from build123d import *

# Parameters (mm, degrees)
SKETCH1_R                = 2.5
BASE_EXTRUDE_DEPTH       = 1
PROCESS_BENDS1_START     = 0.384624116
PROCESS_BENDS1_OUTLINE_W = 60
PROCESS_BENDS1_OUTLINE_H = 1
PROCESS_BENDS1_DEPTH     = 29.615375884
PROCESS_BENDS1_START_2   = -1.84192973
PROCESS_BENDS1_2_DEPTH   = 3.226553846
PROCESS_BENDS1_START_3   = -30
PROCESS_BENDS1_3_DEPTH   = 61
PROCESS_BENDS1_4_DEPTH   = 60


with BuildPart() as part:
    # Sketch1 → Base-Extrude (new body)
    with BuildSketch(Plane.XY):
        with BuildLine():
            Line((14, 18.25), (28, 18.25))
            ThreePointArc((28, 18.25), (29.414213562, 18.835786438), (30, 20.25))
            Line((30, 20.25), (30, 20.725859478))
            ThreePointArc((30, 20.725859478), (29.686782892, 21.800458695), (28.845236523, 22.538475052))
            Line((28.845236523, 22.538475052), (13.245791834, 29.812615574))
            ThreePointArc((13.245791834, 29.812615574), (12.833434539, 29.952592014), (12.400555311, 30))
            Line((12.400555311, 30), (-286, 30))
            ThreePointArc((-286, 30), (-288.828427125, 28.828427125), (-290, 26))
            Line((-290, 26), (-290, -26))
            ThreePointArc((-290, -26), (-288.828427125, -28.828427125), (-286, -30))
            Line((-286, -30), (12.400555311, -30))
            ThreePointArc((12.400555311, -30), (12.833434539, -29.952592014), (13.245791834, -29.812615574))
            Line((13.245791834, -29.812615574), (28.845236523, -22.538475052))
            ThreePointArc((28.845236523, -22.538475052), (29.686782892, -21.800458695), (30, -20.725859478))
            Line((30, -20.725859478), (30, -20.25))
            ThreePointArc((30, -20.25), (29.414213562, -18.835786438), (28, -18.25))
            Line((28, -18.25), (14, -18.25))
            ThreePointArc((14, -18.25), (8.75, -13), (14, -7.75))
            Line((14, -7.75), (28, -7.75))
            ThreePointArc((28, -7.75), (29.414213562, -7.164213562), (30, -5.75))
            Line((30, -5.75), (30, 5.75))
            ThreePointArc((30, 5.75), (29.414213562, 7.164213562), (28, 7.75))
            Line((28, 7.75), (14, 7.75))
            ThreePointArc((14, 7.75), (8.75, 13), (14, 18.25))
        make_face()
        with Locations((-283, 0)):
            Circle(SKETCH1_R, mode=Mode.SUBTRACT)
    extrude(amount=BASE_EXTRUDE_DEPTH)

    # Process-Bends1: read off the stored shape, not the designer's step
    # Process-Bends1 outline → Process-Bends1 (cut)
    with BuildSketch(Plane.YZ.offset(PROCESS_BENDS1_START)):
        with Locations((0, 0.5)):
            Rectangle(PROCESS_BENDS1_OUTLINE_W, PROCESS_BENDS1_OUTLINE_H)
    extrude(amount=PROCESS_BENDS1_DEPTH, mode=Mode.SUBTRACT)

    # Process-Bends1 2 outline → Process-Bends1 2 (add)
    with BuildSketch(Plane.YZ.offset(PROCESS_BENDS1_START_2)):
        with BuildLine():
            ThreePointArc((18.25, 15.384624116), (13, 10.134624116), (7.75, 15.384624116))
            Line((7.75, 15.384624116), (7.75, 29.384624116))
            ThreePointArc((7.75, 29.384624116), (7.164213562, 30.798837678), (5.75, 31.384624116))
            Line((5.75, 31.384624116), (-5.75, 31.384624116))
            ThreePointArc((-5.75, 31.384624116), (-7.164213562, 30.798837678), (-7.75, 29.384624116))
            Line((-7.75, 29.384624116), (-7.75, 15.384624116))
            ThreePointArc((-7.75, 15.384624116), (-13, 10.134624116), (-18.25, 15.384624116))
            Line((-18.25, 15.384624116), (-18.25, 29.384624116))
            ThreePointArc((-18.25, 29.384624116), (-18.835786438, 30.798837678), (-20.25, 31.384624116))
            Line((-20.25, 31.384624116), (-20.725859478, 31.384624116))
            ThreePointArc((-20.725859478, 31.384624116), (-21.800458695, 31.071407008), (-22.538475052, 30.229860639))
            Line((-22.538475052, 30.229860639), (-29.812615574, 14.63041595))
            ThreePointArc((-29.812615574, 14.63041595), (-29.952592014, 14.218058655), (-30, 13.785179427))
            Line((-30, 13.785179427), (-30, 1))
            Line((-30, 1), (30, 1))
            Line((30, 1), (30, 13.785179427))
            ThreePointArc((30, 13.785179427), (29.952592014, 14.218058655), (29.812615574, 14.63041595))
            Line((29.812615574, 14.63041595), (22.538475052, 30.229860639))
            ThreePointArc((22.538475052, 30.229860639), (21.800458695, 31.071407008), (20.725859478, 31.384624116))
            Line((20.725859478, 31.384624116), (20.25, 31.384624116))
            ThreePointArc((20.25, 31.384624116), (18.835786438, 30.798837678), (18.25, 29.384624116))
            Line((18.25, 29.384624116), (18.25, 15.384624116))
        make_face()
    extrude(amount=PROCESS_BENDS1_2_DEPTH)

    # Process-Bends1 3 outline → Process-Bends1 3 (cut)
    with BuildSketch(Plane(origin=(0, 0, 0), x_dir=(1, 0, 0), z_dir=(0, 1, 0)).offset(PROCESS_BENDS1_START_3)):
        with BuildLine():
            ThreePointArc((-2.615375884, 0), (0.213051241, -1.171572875), (1.384624116, -4))
            Line((1.384624116, -4), (1.384624116, -1))
            Line((1.384624116, -1), (0.384624116, -1))
            Line((0.384624116, -1), (0.384624116, 0))
            Line((0.384624116, 0), (-2.615375884, 0))
        make_face()
        with BuildLine():
            Line((0.384624116, -31.384624116), (0.384624116, -4))
            ThreePointArc((0.384624116, -4), (-0.236264867, -2.172479612), (-1.84192973, -1.101417407))
            Line((-1.84192973, -1.101417407), (-1.84192973, -31.384624116))
            Line((-1.84192973, -31.384624116), (0.384624116, -31.384624116))
        make_face()
    extrude(amount=PROCESS_BENDS1_3_DEPTH, mode=Mode.SUBTRACT)

    # Process-Bends1 4 outline → Process-Bends1 4 (add)
    with BuildSketch(Plane(origin=(0, 0, 0), x_dir=(1, 0, 0), z_dir=(0, 1, 0)).offset(PROCESS_BENDS1_START_3)):
        with BuildLine():
            ThreePointArc((-2.615375884, -1), (-2.22534241, -1.025462408), (-1.84192973, -1.101417407))
            Line((-1.84192973, -1.101417407), (-1.84192973, -1))
            Line((-1.84192973, -1), (-2.615375884, -1))
        make_face()
    extrude(amount=PROCESS_BENDS1_4_DEPTH)


solid = part.part
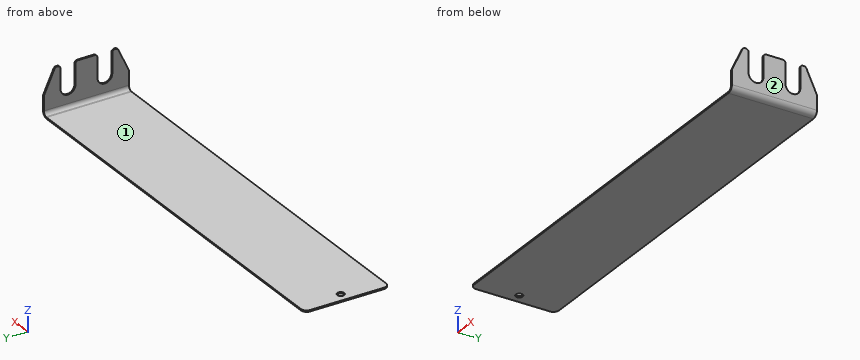
CAD build for the part. Positions are in the model's coordinates, mm. Face numbers are marked on the shaded views. A direction names the side the tool comes from. Give positions to 0.01 mm unless a question says otherwise; leave off trailing zeros. Write each loop counter-clockwise with the first axis right and the second up, starting at its lowest first coordinate (ties: lowest second). Pieces come first, ordered by that corner, then holes. Notation, with made-up numbers: (67.5, -24) -> (79.5, -24) arc R19 cw to (79.5, 11) -> close; hole circle Ø10 at (42, 37.25). An arc over 180 degrees is marked (long way). Return JSON: item names as keys, results as strings.
Item 1: Band-saw the part on A-A (x = -283). List the corners of the cut face in (y, z), then the cut area to 3 significant figures.
Answer below:
{"outline": "(-30, 0) -> (-2.5, 0) -> (-2.5, 1) -> (-30, 1) -> close; (2.5, 0) -> (30, 0) -> (30, 1) -> (2.5, 1) -> close", "area": "55.0 mm2"}
Item 2: Drill centre lines: probe 1 along Y at (x, z) = (-283, 0.7); probe 2 along X at (y, z) = (-2.5, 18); probe 3 along Z at (x, y) = (-186, -8). Where is each one in solid material? Low to high.
Answer below:
{"probe 1": "y = -30 to -2.5, 2.5 to 30", "probe 2": "x = 0.38 to 1.38", "probe 3": "z = 0 to 1"}
Item 3: Band-saw the part on C-C (z = 26.5). List the corners of the cut face in (x, y), then the cut area to 3 significant figures.
Answer below:
{"outline": "(0.38, -24.28) -> (1.38, -24.28) -> (1.38, -18.25) -> (0.38, -18.25) -> close; (0.38, -7.75) -> (1.38, -7.75) -> (1.38, 7.75) -> (0.38, 7.75) -> close; (0.38, 18.25) -> (1.38, 18.25) -> (1.38, 24.28) -> (0.38, 24.28) -> close", "area": "27.6 mm2"}
Item 4: Drop flat-ended pins along their axis: pin 1 (0.8 mm diameter, centred on x = 1, z = 21, fed in from -Y); pin 2 (1.1 mm diameter, centred on x = 1, z = 23.5, fed in from +Y); pin 3 (5 mm diameter, centred on y = -23.5, z = 24.5, fed in from -X). Give the stop position or say it passes through.
Answer below:
{"pin 1": "stops at y = -27.03", "pin 2": "stops at y = 25.93", "pin 3": "stops at x = 0.38"}
Item 5: Tool access for the marked faces 1 and 2: list every direction of +Z, -Z, +X, -X, +Y, -Y with a clear straight run to the whole face (end or side of a thin tool).
Answer below:
{"face 1": "+Z, -X, +Y, -Y", "face 2": "+Z, -Z, +X, +Y, -Y"}
Item 6: Band-saw the part on B-B (y = 0). List the corners of the cut face in (x, z), then the cut area to 3 significant figures.
Answer below:
{"outline": "(-290, 0) -> (-285.5, 0) -> (-285.5, 1) -> (-290, 1) -> close; (-280.5, 0) -> (-2.62, 0) arc R4 ccw to (1.38, 4) -> (1.38, 31.38) -> (0.38, 31.38) -> (0.38, 4) arc R3 cw to (-2.62, 1) -> (-280.5, 1) -> close", "area": "315 mm2"}
Item 7: Band-saw the part on D-D (y = -13). List the corners of the cut face in (x, z).
Answer below:
{"outline": "(-290, 0) -> (-2.62, 0) arc R4 ccw to (1.38, 4) -> (1.38, 10.13) -> (0.38, 10.13) -> (0.38, 4) arc R3 cw to (-2.62, 1) -> (-290, 1) -> close"}
